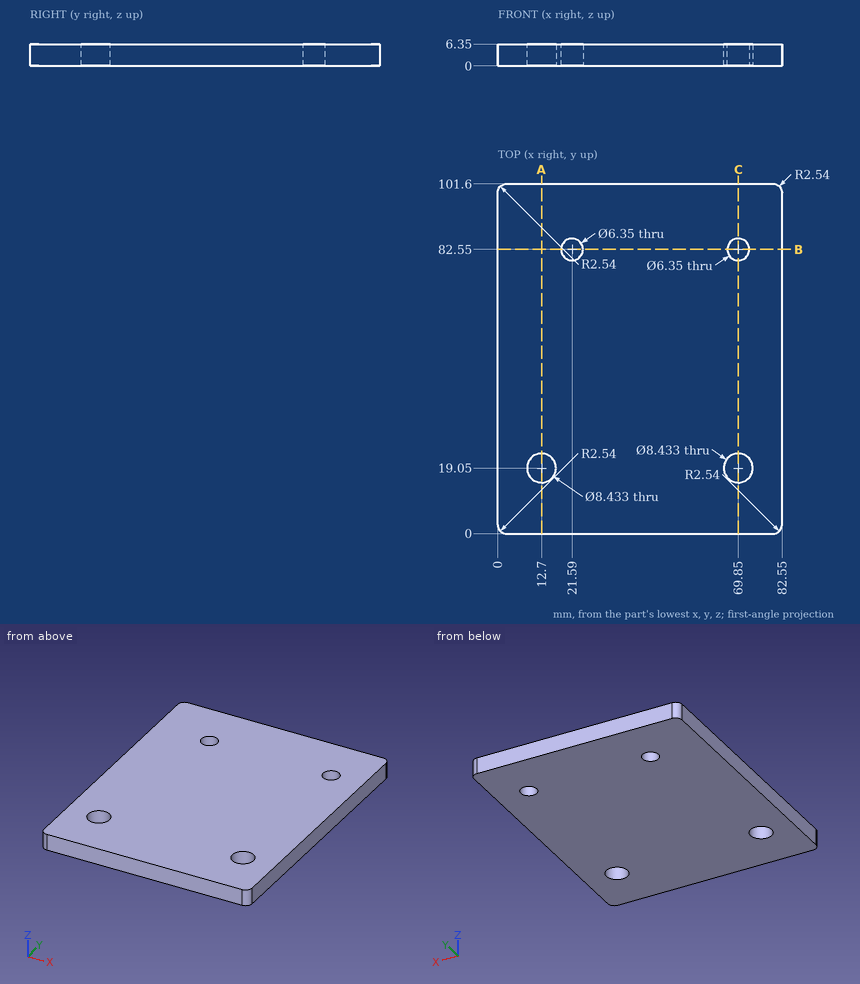
Could you check a few things on this drawing? It's one solid part, dimensions in mm from its lowest x, y, z. Give positions to 0.01 mm unless a question says otherwise; leave off trailing zeros. Order: outer loops, then holes, each group sorted by start corner. A loop starts at its lowest first (then second) coordinate and runs counter-clockwise, first axis right, second up.
1. Suppose I cut it at B-B (y = 82.55). Write out the boundary of the cut face in (x, z) (3 decimals).
Answers below:
outline: (0, 0) - (18.415, 0) - (18.415, 6.35) - (0, 6.35) - close; (24.765, 0) - (66.675, 0) - (66.675, 6.35) - (24.765, 6.35) - close; (73.025, 0) - (82.55, 0) - (82.55, 6.35) - (73.025, 6.35) - close
2. I need wall thicknesses on L1, parallel to Y at x = 12.7, z = 4.5; L2, parallel to Y at x = 21, z = 4.5; L3, parallel to X at y = 16.5, z = 3.5. Which ranges of each line are inside material? Lowest first, please.
Answers below:
L1: y = 0 to 14.83, 23.27 to 101.6
L2: y = 0 to 79.43, 85.67 to 101.6
L3: x = 0 to 9.34, 16.06 to 66.49, 73.21 to 82.55
3. Suppose I cut it at A-A (x = 12.7). Write out the boundary of the cut face in (y, z), plus the area to 3 significant figures.
Answers below:
outline: (0, 0) - (14.83, 0) - (14.83, 6.35) - (0, 6.35) - close; (23.27, 0) - (101.6, 0) - (101.6, 6.35) - (23.27, 6.35) - close
area: 592 mm2
4. Suppose I cut it at C-C (x = 69.85). State how many separate pieces and enclosed holes the cut face has, plus the area to 3 significant figures.
Answers below:
separate pieces: 3
enclosed holes: 0
area: 551 mm2
